from build123d import *

# Parameters (mm, degrees)
SKETCH1_R           = 7.5
SKETCH1_R_2         = 3
BOSS_EXTRUDE1_DEPTH = 3
FILLET1_R           = 0.3


with BuildPart() as part:
    # Sketch1 → Boss-Extrude1 (new body, symmetric)
    with BuildSketch(Plane(origin=(0, 0, 0), x_dir=(1, 0, 0), z_dir=(0, 1, 0))):
        Circle(SKETCH1_R)
        Circle(SKETCH1_R_2, mode=Mode.SUBTRACT)
    extrude(amount=BOSS_EXTRUDE1_DEPTH, both=True)

    # Fillet1
    fillet1_edges = [part.edges().sort_by_distance(p)[0] for p in [
        (-7.5, -3, 0),
        (-7.5, 3, 0),
        (-3, -3, 0),
        (-3, 3, 0),
    ]]
    fillet(fillet1_edges, radius=FILLET1_R)


solid = part.part
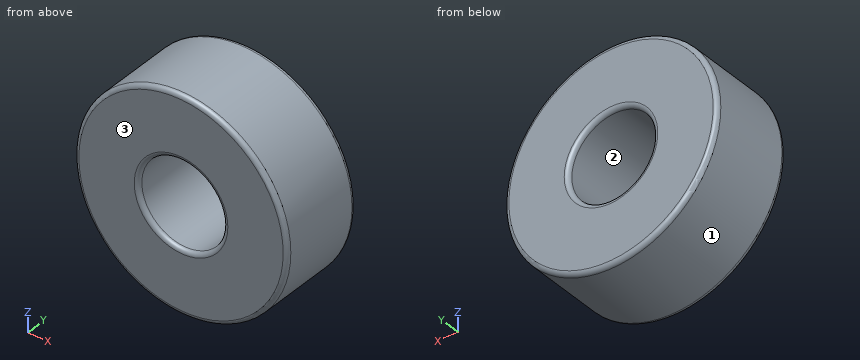
Could you check a few things on this model? Use its own coordinates, in mm. Face numbers are marked on the shaded views. Round coordinates to 2 decimals unless told otherwise and drop trailing zeros. Order: outer loops, then holes, each group sorted by start corner. A loop starts at its lowest first (then second) coordinate and runs counter-clockwise, first axis right, second up.
(1) Imagine slicing it at A-A (z = 0). Write out the boundary of the cut face in (x, y), plus the area to 3 significant figures.
Response values:
outline: (-7.5, -2.7) arc R0.3 ccw to (-7.2, -3) - (-3.3, -3) arc R0.3 ccw to (-3, -2.7) - (-3, 2.7) arc R0.3 ccw to (-3.3, 3) - (-7.2, 3) arc R0.3 ccw to (-7.5, 2.7) - close; (3, -2.7) arc R0.3 ccw to (3.3, -3) - (7.2, -3) arc R0.3 ccw to (7.5, -2.7) - (7.5, 2.7) arc R0.3 ccw to (7.2, 3) - (3.3, 3) arc R0.3 ccw to (3, 2.7) - close
area: 53.8 mm2
(2) Imagine slicing it at C-C (y = 2). Write out the boundary of the cut face in (x, z), plus the area to 3 significant figures.
Response values:
outline: circle Ø15 at (0, 0); hole circle Ø6 at (0, 0)
area: 148 mm2
(3) If we mould it in two halves opening along X, with no side actions, what happens to the marked faces 1, 2 and 3? For each: released by +X, released by -X, zero draft, split by the parting line, or undercut.
Response values:
face 1: split by the parting line
face 2: undercut
face 3: zero draft
(4) I'm going to push flat-ended pins straight in: pin 1 (2 mm diameter, centred on y = -1.5, z = 3, fed in from -X); pin 2 (1 mm diameter, centred on x = 5, y = -1.5, fed in from -Z); pin 3 (3 mm diameter, centred on x = 3.5, y = -1, fed in from +Z). Where does each tip first touch, or does it pass through?
Response values:
pin 1: stops at x = -7.23
pin 2: stops at z = -6
pin 3: stops at z = 7.23
(5) Imagine slicing it at B-B (x = 0). Write out the boundary of the cut face in (y, z), plus the area to 3 significant figures.
Response values:
outline: (-3, -7.2) arc R0.3 ccw to (-2.7, -7.5) - (2.7, -7.5) arc R0.3 ccw to (3, -7.2) - (3, -3.3) arc R0.3 ccw to (2.7, -3) - (-2.7, -3) arc R0.3 ccw to (-3, -3.3) - close; (-3, 3.3) arc R0.3 ccw to (-2.7, 3) - (2.7, 3) arc R0.3 ccw to (3, 3.3) - (3, 7.2) arc R0.3 ccw to (2.7, 7.5) - (-2.7, 7.5) arc R0.3 ccw to (-3, 7.2) - close
area: 53.8 mm2
(6) Please list where these lines run through material, in increasing order: line 1 along X through (y, z) = (1.2, 0); line 2 along X through (y, z) = (-0.25, -1.5).
Response values:
line 1: x = -7.5 to -3, 3 to 7.5
line 2: x = -7.35 to -2.6, 2.6 to 7.35
